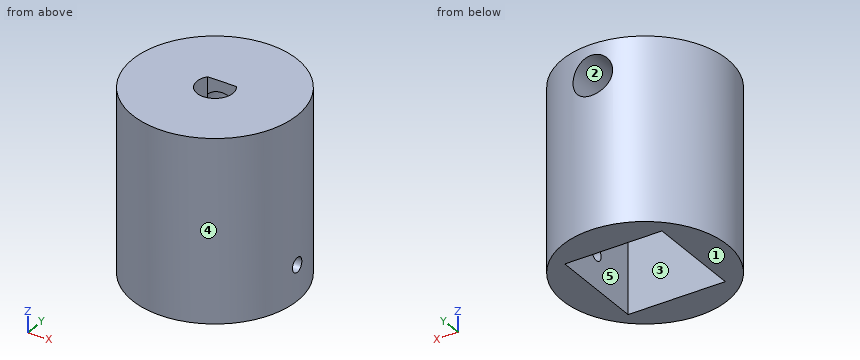
```python
from build123d import *
from build123d.topology import SkipClean

# Parameters (mm, degrees)
BOSS_EXTRUDE1_DEPTH = 9.8
SKETCH2_R           = 9.925
BOSS_EXTRUDE2_DEPTH = 7
SKETCH3_W           = 13.5
SKETCH3_H           = 13.5
CUT_EXTRUDE1_DEPTH  = 5
SKETCH4_R           = 5
BOSS_EXTRUDE3_DEPTH = 8.5
SKETCH5_R           = 1
CUT_EXTRUDE2_DEPTH  = 10.5
SKETCH7_W           = 3.5
SKETCH7_H           = 8.12
CUT_EXTRUDE4_DEPTH  = 10.5
SKETCH9_R           = 9.925
SKETCH9_R_2         = 5
BOSS_EXTRUDE4_DEPTH = 8.5
SKETCH14_R          = 11.46
SKETCH14_R_2        = 9.925
BOSS_EXTRUDE5_DEPTH = 15.5
SKETCH6_R           = 2.75
CUT_EXTRUDE3_DEPTH  = 13.5
CUT_EXTRUDE5_DEPTH  = 21


with BuildPart() as part:
    # Sketch1 → Boss-Extrude1 (new body)
    # profile 1 of 5: a face of its own
    with BuildSketch(Plane.XY):
        with BuildLine():
            Line((17.06, 4.06), (10.716715915, 4.06))
            ThreePointArc((10.716715915, 4.06), (-11.46, 0), (10.716715915, -4.06))
            Line((10.716715915, -4.06), (17.06, -4.06))
            Line((17.06, -4.06), (17.06, 4.06))
        make_face()
        with BuildLine():
            Line((-5.14952425, -6.75), (-6.75, -6.75))
            Line((-6.75, -6.75), (-6.75, -5.14952425))
            ThreePointArc((-6.75, -5.14952425), (-8.49, 0), (-6.75, 5.14952425))
            Line((-6.75, 5.14952425), (-6.75, 6.75))
            Line((-6.75, 6.75), (-5.14952425, 6.75))
            ThreePointArc((-5.14952425, 6.75), (0, 8.49), (5.14952425, 6.75))
            Line((5.14952425, 6.75), (6.75, 6.75))
            Line((6.75, 6.75), (6.75, 5.14952425))
            ThreePointArc((6.75, 5.14952425), (8.49, 0), (6.75, -5.14952425))
            Line((6.75, -5.14952425), (6.75, -6.75))
            Line((6.75, -6.75), (5.14952425, -6.75))
            ThreePointArc((5.14952425, -6.75), (0, -8.49), (-5.14952425, -6.75))
        make_face(mode=Mode.SUBTRACT)
    # profile 2 of 5: a face of its own
    with BuildSketch(Plane.XY):
        with BuildLine():
            ThreePointArc((5.14952425, 6.75), (0, 8.49), (-5.14952425, 6.75))
            Line((-5.14952425, 6.75), (5.14952425, 6.75))
        make_face()
    # profile 3 of 5: a face of its own
    with BuildSketch(Plane.XY):
        with BuildLine():
            ThreePointArc((-6.75, 5.14952425), (-8.49, 0), (-6.75, -5.14952425))
            Line((-6.75, -5.14952425), (-6.75, 5.14952425))
        make_face()
    # profile 4 of 5: a face of its own
    with BuildSketch(Plane.XY):
        with BuildLine():
            Line((6.75, 5.14952425), (6.75, -5.14952425))
            ThreePointArc((6.75, -5.14952425), (8.49, 0), (6.75, 5.14952425))
        make_face()
    # profile 5 of 5: a face of its own
    with BuildSketch(Plane.XY):
        with BuildLine():
            Line((5.14952425, -6.75), (-5.14952425, -6.75))
            ThreePointArc((-5.14952425, -6.75), (0, -8.49), (5.14952425, -6.75))
        make_face()
    extrude(amount=BOSS_EXTRUDE1_DEPTH)

    # Sketch2 → Boss-Extrude2 (add)
    with BuildSketch(Plane.XY.offset(9.8)):
        Circle(SKETCH2_R)
    extrude(amount=BOSS_EXTRUDE2_DEPTH)

    # Sketch3 → Cut-Extrude1 (cut)
    with BuildSketch(Plane(origin=(0, 0, 9.8), x_dir=(-1, 0, 0), z_dir=(0, 0, -1))):
        Rectangle(SKETCH3_W, SKETCH3_H)
    extrude(amount=-CUT_EXTRUDE1_DEPTH, mode=Mode.SUBTRACT)

    # Sketch4 → Boss-Extrude3 (add)
    with BuildSketch(Plane.XY.offset(16.8)):
        Circle(SKETCH4_R)
        with BuildLine():
            Line((2, 1.5), (-2, 1.5))
            ThreePointArc((-2, 1.5), (0, -2.5), (2, 1.5))
        make_face(mode=Mode.SUBTRACT)
    extrude(amount=BOSS_EXTRUDE3_DEPTH)

    # Sketch5 → Cut-Extrude2 (cut)
    with BuildSketch(Plane(origin=(17.06, 0, 0), x_dir=(0, 0, -1), z_dir=(1, 0, 0))):
        with Locations(Location((-4.9, 0, 0), (0, 0, 90))):
            Circle(SKETCH5_R)
    extrude(amount=-CUT_EXTRUDE2_DEPTH, mode=Mode.SUBTRACT)

    # Sketch7 → Cut-Extrude4 (cut)
    with BuildSketch(Plane(origin=(0, 0, 0), x_dir=(-1, 0, 0), z_dir=(0, 0, -1))):
        with Locations((-15.31, 0)):
            Rectangle(SKETCH7_W, SKETCH7_H)
    extrude(amount=-CUT_EXTRUDE4_DEPTH, mode=Mode.SUBTRACT)

    # Sketch9 → Boss-Extrude4 (add)
    with BuildSketch(Plane.XY.offset(16.8)):
        Circle(SKETCH9_R)
        Circle(SKETCH9_R_2, mode=Mode.SUBTRACT)
    extrude(amount=BOSS_EXTRUDE4_DEPTH)

    # Sketch14 → Boss-Extrude5 (add)
    with BuildSketch(Plane.XY.offset(9.8)):
        with Locations(Location((0, 0, 0), (0, 0, 339.250937201))):
            Circle(SKETCH14_R)
        Circle(SKETCH14_R_2, mode=Mode.SUBTRACT)
    extrude(amount=BOSS_EXTRUDE5_DEPTH)

    # Sketch6 → Cut-Extrude3 (cut)
    with BuildSketch(Plane.XZ.offset(-1.5)):
        with Locations(Location((0, 21.05, 0), (0, 0, 270))):
            Circle(SKETCH6_R)
    extrude(amount=-CUT_EXTRUDE3_DEPTH, mode=Mode.SUBTRACT)

    # Sketch15 → Cut-Extrude5 (cut)
    with SkipClean():  # the faces are left unmerged after this step: merging them gives an invalid solid
        with BuildSketch(Plane(origin=(0, 0, 0), x_dir=(-1, 0, 0), z_dir=(0, 0, -1))):
            with BuildLine():
                ThreePointArc((-10.716715915, -4.06), (-11.46, 0), (-10.716715915, 4.06))
                Line((-10.716715915, 4.06), (-13.56, 4.06))
                Line((-13.56, 4.06), (-13.56, -4.06))
                Line((-13.56, -4.06), (-10.716715915, -4.06))
            make_face()
        extrude(amount=-CUT_EXTRUDE5_DEPTH, mode=Mode.SUBTRACT)


solid = part.part
```
Design review of the part built by this model. Coordinates are the model's own, in mm. Face numbers are marked on the shaded views. A direction names the side the tool comes from. Give positions to 0.01 mm unless a question says otherwise; leave off trailing zeros. Write each loop counter-clockwise with the first axis right and the second up, starting at its lowest first coordinate (ties: lowest second). Pieces come first, ordered by that corner, then holes. Notation, with made-up numbers: (84.5, 83) - (96.5, 83) arc R26 ccw to (96.5, 121) - close; hole circle Ø8 at (82.25, 29). An arc over 180 degrees is marked (long way). Return JSON: item names as keys, results as strings. Group by question number.
(1) Insertion check: pin 1 (6 mm diameter, centred on x = 5.5, z = 6.5, fed in from -Y); pin 2 (1.5 mm diameter, centred on x = -1, y = -2, fed in from -Z); pin 3 (8 mm diameter, centred on x = 0, y = 0, fed in from +Z); pin 4 (8 mm diameter, centred on y = 8, z = 22.5, fed in from -X). Each pin has a flat end and moves straight along its axis. Give the tip position at first contact, or say it passes through.
(2) We need section A-A, the plane y = 0. Give the boundary of the cut face in (x, z), then the cut area to 3 significant figures.
(3) We need section B-B, the plane x = 0. Give the boundary of the cut face in (y, z), then the cut area to 3 significant figures.
(4) To check wall thickness, follow probe 1 along X at (y, z) = (0, 21.75); probe 2 along Z at (x, y) = (0, 6); probe 3 along Z at (x, y) = (9.35, 0). State the ranges of each line that lie inside material, in increasing order.
(5) We need section D-D, the plane z = 4.9. Give the boundary of the cut face in (x, y).
(6) We need section C-C, the plane y = 3.5. Give the boundary of the cut face in (x, z).
(7) Mouldability with a two-part tool opening along Z and no side actions: class the marked faces 1, 2 and 3 as +Z half, -Z half, draft (parallel to the pull), parting line (faces both ways), or undercut.
(8) Machinability: for the marked faces 4 and 5, which of the approach directions +Z, -Z, +X, -X, +Y, -Y give a long, thin tool a straight path to every point of the face, cutting with its end or side? Answer none if there is none.
Reported:
{
 "1": {"pin 1": "stops at y = -11.18", "pin 2": "stops at z = 14.8", "pin 3": "stops at z = 25.3", "pin 4": "stops at x = -10.74"},
 "2": {"outline": "(-11.46, 0) - (-6.75, 0) - (-6.75, 14.8) - (6.75, 14.8) - (6.75, 5.9) - (11.46, 5.9) - (11.46, 25.3) - (2.5, 25.3) - (2.5, 16.8) - (-2.5, 16.8) - (-2.5, 25.3) - (-11.46, 25.3) - close; (6.75, 0) - (11.46, 0) - (11.46, 3.9) - (6.75, 3.9) - close", "area": "328 mm2"},
 "3": {"outline": "(-11.46, 0) - (-6.75, 0) - (-6.75, 14.8) - (6.75, 14.8) - (6.75, 0) - (11.46, 0) - (11.46, 18.3) - (1.5, 18.3) - (1.5, 16.8) - (-2.5, 16.8) - (-2.5, 25.3) - (-11.46, 25.3) - close; (1.5, 23.8) - (11.46, 23.8) - (11.46, 25.3) - (1.5, 25.3) - close", "area": "291 mm2"},
 "4": {"probe 1": "x = -11.46 to -2.5, 2.5 to 11.46", "probe 2": "z = 14.8 to 18.3, 23.8 to 25.3", "probe 3": "z = 0 to 3.9, 5.9 to 25.3"},
 "5": {"outline": "(-6.75, -6.75) - (-6.75, 6.75) - (6.75, 6.75) - (6.75, 1) - (11.42, 1) arc R11.46 ccw (long way) to (11.42, -1) - (6.75, -1) - (6.75, -6.75) - close"},
 "6": {"outline": "(-10.91, 0) - (-6.75, 0) - (-6.75, 14.8) - (6.75, 14.8) - (6.75, 0) - (10.91, 0) - (10.91, 25.3) - (-10.91, 25.3) - close; hole circle Ø5.5 at (0, 21.05)"},
 "7": {"face 1": "-Z half", "face 2": "undercut", "face 3": "draft"},
 "8": {"face 4": "+Z, -Z", "face 5": "-Z"}
}
